Input: part model. Units: mm. Frame: model coordinates. Give positions to 0.01 mm unless a question says otherwise; leave off trailing zeros. Loops run counter-clockwise (first coordinate to the right, second up) from the corner with the lowest first, then second, coordinate; pieces in that order, holes last. Notation, with made-up numbers: M -27.5,21 L 9.5,21 A19 ccw 9.5,39 Z; hole C 67.5,-14.75 d5. An arc over 180 degrees is marked long. One line per item, written item: value. Start each with the question number.
(1) Pin query (flat end, axial travel): P1, Ø5, axis at x = 65, z = 70, coming from the -Y side; P2, Ø3.5, axis at x = 65, z = 10, coming from the -Y side. Return the tip coordinate at first contact, or that it passes through.
(2) Ray query, line 1 along X through (y, z) = (2.1, 60); line 2 along X through (y, z) = (1.3, 70); line 3 along Z through (x, y) = (63.5, 1.7). Return the intervals inside material, ascending. Write a range as from..to.
(3) Section C-C on y = 0.85. State how many separate pieces and enclosed holes the cut face has, plus the area to 3 significant figures.
(4) Section A-A on x = 65. Output: boundary loops of the cut face in (y, z).
(5) Section D-D on x = 35. Output: boundary loops of the cut face in (y, z).
(6) Section B-B on z = 10. Output: boundary loops of the cut face in (x, y), plus the area to 4 significant figures.
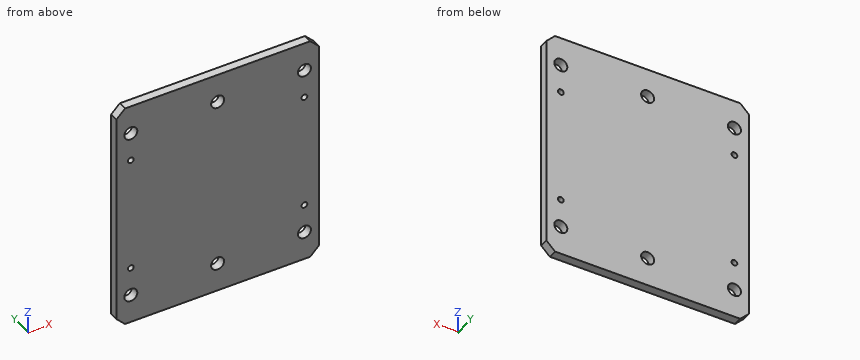
```python
from build123d import *

# Parameters (mm, degrees)
ESQUISSE1_W             = 70
ESQUISSE1_H             = 12
BOSS_EXTRU_1_DEPTH      = 80
ESQUISSE2_W             = 12
ESQUISSE2_H             = 6
ENL_V_MAT_EXTRU_1_DEPTH = 107.976632963
ESQUISSE4_R             = 2.25
ENL_V_MAT_EXTRU_3_DEPTH = 107.976632963
ESQUISSE5_W             = 12
ESQUISSE5_H             = 10
BOSS_EXTRU_2_DEPTH      = 6
CHANFREIN1_SIZE         = 3
ESQUISSE6_R             = 1
ENL_V_MAT_EXTRU_4_DEPTH = 12
ESQUISSE8_W             = 70
ESQUISSE8_H             = 9
ENL_V_MAT_EXTRU_8_DEPTH = 80


with BuildPart() as part:
    # Esquisse1 → Boss.-Extru.1 (new body)
    with BuildSketch(Plane.XY):
        with Locations((35, 6)):
            Rectangle(ESQUISSE1_W, ESQUISSE1_H)
    extrude(amount=BOSS_EXTRU_1_DEPTH)

    # Esquisse2 → Enlèv. mat.-Extru.1 (cut, through all)
    with BuildSketch(Plane.XY.offset(80)):
        with Locations((52.5, 9)):
            Rectangle(ESQUISSE2_W, ESQUISSE2_H)
        with Locations((17.5, 9)):
            Rectangle(ESQUISSE2_W, ESQUISSE2_H)
    extrude(amount=-ENL_V_MAT_EXTRU_1_DEPTH, mode=Mode.SUBTRACT)

    # Esquisse4 → Enlèv. mat.-Extru.3 (cut, through all)
    with BuildSketch(Plane(origin=(0, 12, 0), x_dir=(1, 0, 0), z_dir=(0, 1, 0))):
        with Locations(Location((5, -10, 0), (0, 0, 270))):
            Circle(ESQUISSE4_R)
        with Locations(Location((65, -70, 0), (0, 0, 270))):
            Circle(ESQUISSE4_R)
        with Locations(Location((65, -10, 0), (0, 0, 90))):
            Circle(ESQUISSE4_R)
        with Locations(Location((5, -70, 0), (0, 0, 90))):
            Circle(ESQUISSE4_R)
        with Locations(Location((35, -10, 0), (0, 0, 270))):
            Circle(ESQUISSE4_R)
        with Locations(Location((35, -70, 0), (0, 0, 270))):
            Circle(ESQUISSE4_R)
    extrude(amount=-ENL_V_MAT_EXTRU_3_DEPTH, mode=Mode.SUBTRACT)

    # Esquisse5 → Boss.-Extru.2 (add)
    with BuildSketch(Plane(origin=(0, 12, 0), x_dir=(1, 0, 0), z_dir=(0, 1, 0))):
        with Locations((17.5, -75)):
            Rectangle(ESQUISSE5_W, ESQUISSE5_H)
        with Locations((52.5, -75)):
            Rectangle(ESQUISSE5_W, ESQUISSE5_H)
        with Locations((52.5, -5)):
            Rectangle(ESQUISSE5_W, ESQUISSE5_H)
        with Locations((17.5, -5)):
            Rectangle(ESQUISSE5_W, ESQUISSE5_H)
    extrude(amount=-BOSS_EXTRU_2_DEPTH)

    # Chanfrein1
    chanfrein1_edges = [part.edges().sort_by_distance(p)[0] for p in [
        (70, 6, 80),
        (0, 6, 80),
        (70, 6, 0),
        (0, 6, 0),
    ]]
    chamfer(chanfrein1_edges, length=CHANFREIN1_SIZE)

    # Esquisse6 → Enlèv. mat.-Extru.4 (cut)
    with BuildSketch(Plane(origin=(0, 12, 0), x_dir=(1, 0, 0), z_dir=(0, 1, 0))):
        with Locations(Location((5, -20, 0), (0, 0, 270))):
            Circle(ESQUISSE6_R)
        with Locations(Location((5, -60, 0), (0, 0, 90))):
            Circle(ESQUISSE6_R)
        with Locations(Location((65, -60, 0), (0, 0, 270))):
            Circle(ESQUISSE6_R)
        with Locations(Location((65, -20, 0), (0, 0, 90))):
            Circle(ESQUISSE6_R)
    extrude(amount=-ENL_V_MAT_EXTRU_4_DEPTH, mode=Mode.SUBTRACT)

    # Esquisse8 → Enlèv. mat.-Extru.8 (cut)
    with BuildSketch(Plane.XY.offset(80)):
        with Locations((35, 7.5)):
            Rectangle(ESQUISSE8_W, ESQUISSE8_H)
    extrude(amount=-ENL_V_MAT_EXTRU_8_DEPTH, mode=Mode.SUBTRACT)


solid = part.part
```
Output values:
1. P1: stops at y = 0
1. P2: passes through
2. line 1: x = 0..4, 6..64, 66..70
2. line 2: x = 0..2.75, 7.25..32.75, 37.25..62.75, 67.25..70
2. line 3: z = 0..8.32, 11.68..68.32, 71.68..80
3. separate pieces: 1
3. enclosed holes: 10
3. area: 5,470 mm²
4. outline: M 0,0 L 3,0 L 3,7.75 L 0,7.75 Z; M 0,12.25 L 3,12.25 L 3,19 L 0,19 Z; M 0,21 L 3,21 L 3,59 L 0,59 Z; M 0,61 L 3,61 L 3,67.75 L 0,67.75 Z; M 0,72.25 L 3,72.25 L 3,80 L 0,80 Z
5. outline: M 0,0 L 3,0 L 3,7.75 L 0,7.75 Z; M 0,12.25 L 3,12.25 L 3,67.75 L 0,67.75 Z; M 0,72.25 L 3,72.25 L 3,80 L 0,80 Z
6. outline: M 0,0 L 2.75,0 L 2.75,3 L 0,3 Z; M 7.25,0 L 32.75,0 L 32.75,3 L 7.25,3 Z; M 37.25,0 L 62.75,0 L 62.75,3 L 37.25,3 Z; M 67.25,0 L 70,0 L 70,3 L 67.25,3 Z
6. area: 169.5 mm²
